from build123d import *

# Parameters (mm, degrees)
SKETCH_1_R           = 42.5
EXTRUDE_7_DEPTH      = 1.5
CUT_EXTRUDE_24_DEPTH = 1.5
CUT_EXTRUDE_25_DEPTH = 1.5
SKETCH_1_14_R        = 1.5
CUT_EXTRUDE_26_DEPTH = 1.5
SKETCH_1_15_R        = 1.5
CUT_EXTRUDE_27_DEPTH = 1.5
SKETCH_1_16_R        = 1.5
CUT_EXTRUDE_28_DEPTH = 1.5
SKETCH_1_17_R        = 1.5
CUT_EXTRUDE_29_DEPTH = 1.5
SKETCH_10_R          = 1.5
CUT_EXTRUDE_31_DEPTH = 98.67420335
SKETCH_11_R          = 6
CUT_EXTRUDE_32_DEPTH = 98.67420335
CUT_EXTRUDE_35_DEPTH = 5
SKETCH_41_W          = 3
SKETCH_41_H          = 50
EXTRUDE_14_DEPTH     = 40
SKETCH_42_W          = 3
SKETCH_42_H          = 50
EXTRUDE_15_DEPTH     = 40


with BuildPart() as part:
    # 草图1 → 凸台-拉伸7 (new, symmetric)
    with BuildSketch(Plane.XY):
        with Locations((20, -37.5)):
            Circle(SKETCH_1_R)
    extrude(amount=EXTRUDE_7_DEPTH, both=True)

    # 草图1<12> → 切除-拉伸24 (cut, symmetric)
    with BuildSketch(Plane.XY):
        with BuildLine():
            ThreePointArc((40, 0), (20, 5), (0, 0))
            Line((0, 0), (40, 0))
        make_face()
    extrude(amount=CUT_EXTRUDE_24_DEPTH, both=True, mode=Mode.SUBTRACT)

    # 草图1<13> → 切除-拉伸25 (cut, symmetric)
    with BuildSketch(Plane.XY):
        with BuildLine():
            Line((40, -75), (0, -75))
            ThreePointArc((0, -75), (20, -80), (40, -75))
        make_face()
    extrude(amount=CUT_EXTRUDE_25_DEPTH, both=True, mode=Mode.SUBTRACT)

    # 草图1<14> → 切除-拉伸26 (cut, symmetric)
    with BuildSketch(Plane.XY):
        with Locations((5, -5)):
            Circle(SKETCH_1_14_R)
    extrude(amount=CUT_EXTRUDE_26_DEPTH, both=True, mode=Mode.SUBTRACT)

    # 草图1<15> → 切除-拉伸27 (cut, symmetric)
    with BuildSketch(Plane.XY):
        with Locations((35, -5)):
            Circle(SKETCH_1_15_R)
    extrude(amount=CUT_EXTRUDE_27_DEPTH, both=True, mode=Mode.SUBTRACT)

    # 草图1<16> → 切除-拉伸28 (cut, symmetric)
    with BuildSketch(Plane.XY):
        with Locations((5, -70)):
            Circle(SKETCH_1_16_R)
    extrude(amount=CUT_EXTRUDE_28_DEPTH, both=True, mode=Mode.SUBTRACT)

    # 草图1<17> → 切除-拉伸29 (cut, symmetric)
    with BuildSketch(Plane.XY):
        with Locations((35, -70)):
            Circle(SKETCH_1_17_R)
    extrude(amount=CUT_EXTRUDE_29_DEPTH, both=True, mode=Mode.SUBTRACT)

    # 草图10 → 切除-拉伸31 (cut, through all)
    with BuildSketch(Plane.XY.offset(1.5)):
        with Locations((20, -15.5)):
            Circle(SKETCH_10_R)
        with Locations((-2, -37.5)):
            Circle(SKETCH_10_R)
        with Locations((42, -37.5)):
            Circle(SKETCH_10_R)
        with Locations((20, -59.5)):
            Circle(SKETCH_10_R)
        with Locations((20, -22.5)):
            Circle(SKETCH_10_R)
        with Locations((5, -37.5)):
            Circle(SKETCH_10_R)
        with Locations((20, -52.5)):
            Circle(SKETCH_10_R)
        with Locations((35, -37.5)):
            Circle(SKETCH_10_R)
    extrude(amount=-CUT_EXTRUDE_31_DEPTH, mode=Mode.SUBTRACT)

    # 草图11 → 切除-拉伸32 (cut, through all)
    with BuildSketch(Plane.XY.offset(1.5)):
        with Locations((20, -37.5)):
            Circle(SKETCH_11_R)
    extrude(amount=-CUT_EXTRUDE_32_DEPTH, mode=Mode.SUBTRACT)

    # 草图19 → 切除-拉伸35 (cut, symmetric)
    with BuildSketch(Plane.XY.offset(1.5)):
        with BuildLine():
            Line((-14.369317712, -62.5), (-14.369317712, -12.5))
            ThreePointArc((-14.369317712, -12.5), (-22.5, -37.5), (-14.369317712, -62.5))
        make_face()
        with BuildLine():
            ThreePointArc((54.369317712, -62.5), (62.5, -37.5), (54.369317712, -12.5))
            Line((54.369317712, -12.5), (54.369317712, -62.5))
        make_face()
    extrude(amount=CUT_EXTRUDE_35_DEPTH, both=True, mode=Mode.SUBTRACT)

    # 草图41 → 凸台-拉伸14 (add)
    with BuildSketch(Plane(origin=(54.369317712, 0, 0), x_dir=(0, 0, -1), z_dir=(1, 0, 0))):
        with Locations((0, -37.5)):
            Rectangle(SKETCH_41_W, SKETCH_41_H)
    extrude(amount=EXTRUDE_14_DEPTH)

    # 草图42 → 凸台-拉伸15 (add)
    with BuildSketch(Plane.ZY.offset(14.369317712)):
        with Locations((0, -37.5)):
            Rectangle(SKETCH_42_W, SKETCH_42_H)
    extrude(amount=EXTRUDE_15_DEPTH)


solid = part.part
Geometry: final body of the model. Coordinates: model frame, mm. A direction names the side the tool comes from. Round coordinates to 2 decimals unless told otherwise and drop trailing zeros. Loops run counter-clockwise (first coordinate to the right, second up) from the corner with the lowest first, then second, coordinate; pieces in that order, holes last. Notation, with made-up numbers: M 16.25,73.5 L 37.25,73.5 A22 cw 37.25,89.5 Z; hole C 43,36 d11. An arc over 180 degrees is marked long. One line per question, with ' | ' between items.
(1) Access query for faces 1 (the flat face through (-34, -62.5, 0)), 2 (the flat face through (-34, -12.5, 0)), 3 (the cylindrical face through (18.89, -21.49, 0.02)), 4 (the flat face through (21, -30, 1.5)), 5 (the flat face through (74, -62.5, 0)). Directions: +Z, -Z, +X, -X, +Y, -Y. A direction counts if a zero-diameter tool reaches every point of the face in a straight line with its end or side. Return the directions, or none.
Check result:
face 1: +Z, -Z, -X, -Y | face 2: +Z, -Z, -X, +Y | face 3: +Z, -Z | face 4: +Z, +X, -X, +Y, -Y | face 5: +Z, -Z, +X, -Y
(2) Pull-direction query (Y, two-part tool) for faces 6 (the cylindrical face through (40.8, -38.4, 0)), 7 (the flat face through (21, -30, -1.5)), 8 (the flat face through (20, 0, 0)); classes: +Y half, -Y half, draft (parallel to the pull), parting line (faces both ways), or undercut.
Check result:
face 6: undercut | face 7: draft | face 8: +Y half
(3) Cut plane B-B on z = 1. Give the number of separate pieces and of enclosed holes in the cut face, plus the area to 3 significant figures.
Check result:
separate pieces: 1 | enclosed holes: 13 | area: 8,650 mm2
(4) Cut plane C-C on x = 5. Return the cut outline in (y, z), plus the area to 3 significant figures.
Check result:
outline: M -75,-1.5 L -71.5,-1.5 L -71.5,1.5 L -75,1.5 Z; M -68.5,-1.5 L -39,-1.5 L -39,1.5 L -68.5,1.5 Z; M -36,-1.5 L -6.5,-1.5 L -6.5,1.5 L -36,1.5 Z; M -3.5,-1.5 L 0,-1.5 L 0,1.5 L -3.5,1.5 Z | area: 198 mm2
(5) Cut plane A-A on y = -52.5. Return the cut outline in (x, z).
Check result:
outline: M -54.37,-1.5 L 18.5,-1.5 L 18.5,1.5 L -54.37,1.5 Z; M 21.5,-1.5 L 94.37,-1.5 L 94.37,1.5 L 21.5,1.5 Z
(6) Material intervals for line 1 along Y through (x, z) = (5, -0.45); line 2 along Y through (x, z) = (20, 0.4); line 3 along X through (y, z) = (-38.5, 0.95), sorted ascending. Write a range as from..to.
Check result:
line 1: y = -75..-71.5, -68.5..-39, -36..-6.5, -3.5..0 | line 2: y = -75..-61, -58..-54, -51..-43.5, -31.5..-24, -21..-17, -14..0 | line 3: x = -54.37..-3.12, -0.88..3.88, 6.12..14.08, 25.92..33.88, 36.12..40.88, 43.12..94.37
(7) Cut plane D-D on y = -37.5. Return the cut outline in (x, z), plus the area to 3 significant figures.
Check result:
outline: M -54.37,-1.5 L -3.5,-1.5 L -3.5,1.5 L -54.37,1.5 Z; M -0.5,-1.5 L 3.5,-1.5 L 3.5,1.5 L -0.5,1.5 Z; M 6.5,-1.5 L 14,-1.5 L 14,1.5 L 6.5,1.5 Z; M 26,-1.5 L 33.5,-1.5 L 33.5,1.5 L 26,1.5 Z; M 36.5,-1.5 L 40.5,-1.5 L 40.5,1.5 L 36.5,1.5 Z; M 43.5,-1.5 L 94.37,-1.5 L 94.37,1.5 L 43.5,1.5 Z | area: 374 mm2
(8) Contact query for flat-ended pins moving along their axis: P1, Ø3.5, axis at x = 20, y = -59.5, coming from the -Z side; P2, Ø1.5, axis at x = 81, z = 0.5, coming from the +Y side; P3, Ø2.5, axis at x = 5, y = -70, coming from the -Z side; P4, Ø1, axis at y = -63.5, z = -0.5, coming from the -X side. Output: stop coordinate, or through.
Check result:
P1: stops at z = -1.5 | P2: stops at y = -12.5 | P3: passes through | P4: stops at x = -14
